from build123d import *

# Parameters (mm, degrees)
F0_R     = 27.5
F0_R_2   = 19
F0_R_3   = 5.5
F1_DEPTH = 100
F2_R     = 20
F3_R     = 18
F4_DEPTH = 60


with BuildPart() as f1:
    # F0 (on Top) → F1 (new body)
    with BuildSketch(Plane.XY):
        Circle(F0_R)
        Circle(F0_R_2, mode=Mode.SUBTRACT)
        Circle(F0_R_2)
        Circle(F0_R_3, mode=Mode.SUBTRACT)
    extrude(amount=F1_DEPTH)

    # F2
    f2_edges = [f1.edges().sort_by_distance(p)[0] for p in [
        (-27.5, 0, 100),
        (-27.5, 0, 0),
    ]]
    fillet(f2_edges, radius=F2_R)


with BuildPart() as f4:
    # F3 (on Top) → F4 (new body)
    with BuildSketch(Plane.XY):
        Circle(F3_R)
    extrude(amount=F4_DEPTH)


with BuildPart() as f1_1:
    add(f1.part)

    # F5: cut F4
    add(f4.part, mode=Mode.SUBTRACT)


solid = f1_1.part
Can you work these out from the model? Positions are in its coordinate system, mm. A direction names the side the tool comes from. Coordinates: 2 decimals unless noted, no trailing zeros. Order: outer loops, then holes, each group sorted by start corner. A loop starts at its lowest first (then second) coordinate and runs counter-clockwise, first axis right, second up. Notation, with made-up numbers: M 17,41 L 65,41 A18 cw 65,71 Z; hole C -27.5,46.25 d11. An arc over 180 degrees is marked long. Write item = value, one per line.
(1) I need wall thicknesses on line 1 along Y through (x, z) = (0, 80.5); line 2 along Y through (x, z) = (0, 37); line 3 along X through (y, z) = (0, 89). Which ranges of each line are inside material? Lowest first, please. Write a range as [from, to].
Results are:
line_1 = [-27.49, -5.5], [5.5, 27.49]
line_2 = [-27.5, -18], [18, 27.5]
line_3 = [-25.36, -5.5], [5.5, 25.36]
(2) If we mould it in two halves opening along X, with no side actions, what happens to faces 3 (the face through (-5.961, -26.846, 49.58)), 4 (the face through (-4, 4, 100)), 5 (the face through (-2.343, 17.847, 31.09))? For each: pulls with the +X half, pulls with the -X half, needs draft (parallel to the pull), parting line crosses it, or undercut.
Results are:
face_3 = parting line crosses it
face_4 = needs draft
face_5 = undercut
(3) Suppose I cut it at B-B on z = 47. Please give me the cut outline in (x, y).
Results are:
outline = C 0,0 d55; hole C 0,0 d36
(4) Suppose I cut it at A-A on z = 66. Please give me the cut outline in (x, y).
Results are:
outline = C 0,0 d55; hole C 0,0 d11
(5) For pin 1 Ø4 at (y, z) = (-14.5, 31.5) entering from +X; pin 2 Ø1.5 at (x, y) = (-15.5, 16) entering from +Z; pin 3 Ø2 at (x, z) = (-4, 55.5) entering from -Y, each with a flat end and sliding along its axis, tell me the tip position at first contact or that it passes through.
Results are:
pin_1 = 24.49
pin_2 = 94.26
pin_3 = -27.34
(6) For faces 1 (the face through (-4, -4, 60)), 2 (the face through (-1.19, -5.37, 79.72)), which set-ups out of +Z, -Z, +X, -X, +Y, -Y let a thin tool reach every point of the face, with its end or its side?
Results are:
face_1 = -Z
face_2 = +Z, -Z
